Can you work these out from the model? Positions are in its coordinate system, mm. Face numbers are marked on the shaded views. Give positions to 0.01 mm unless a question says otherwise; leave off trailing zeros. Order: outer loops, then holes, each group sorted by start corner. A loop starts at its lowest first (then second) coordinate and runs counter-clockwise, first axis right, second up. Notation, with made-up numbers: M 9,1 L 37,1 A9 cw 37,16 Z; hole C 86,19 d6. An arc over 180 degrees is marked long. Answer as a JSON object with one key per item and string values.
```python
from build123d import *

# Parameters (mm, degrees)
SKETCH1_R                = 50
SKETCH1_R_2              = 2.778
BOSS_EXTRUDE1_DEPTH      = 2.5
SKETCH2_W                = 5
SKETCH2_H                = 63.3
BOSS_EXTRUDE2_DEPTH      = 50
FILLET1_R                = 10
SKETCH14_W               = 40.64
SKETCH14_H               = 20.32
CUT_EXTRUDE1_DEPTH       = 30.305745908
F_3_0_3_DIAMETER_HOLE1_D = 3
FILLET1_OF_MIRROR1_R     = 10


with BuildPart() as part:
    # Sketch1 → Boss-Extrude1 (new body, symmetric)
    with BuildSketch(Plane(origin=(0, 0, 0), x_dir=(1, 0, 0), z_dir=(0, 1, 0))):
        Circle(SKETCH1_R)
        Circle(SKETCH1_R_2, mode=Mode.SUBTRACT)
    extrude(amount=BOSS_EXTRUDE1_DEPTH, both=True)

    # Sketch2 → Boss-Extrude2 (add)
    with BuildSketch(Plane(origin=(0, 2.5, 0), x_dir=(1, 0, 0), z_dir=(0, 1, 0))):
        with Locations((-23.194254092, 0)):
            Rectangle(SKETCH2_W, SKETCH2_H)
    boss_extrude2 = extrude(amount=BOSS_EXTRUDE2_DEPTH)

    # Fillet1
    fillet1_edges = [part.edges().sort_by_distance(p)[0] for p in [
        (-23.194254092, 52.5, -31.65),
        (-23.194254092, 52.5, 31.65),
    ]]
    fillet(fillet1_edges, radius=FILLET1_R)

    # Sketch14 → Cut-Extrude1 (cut, through all)
    with BuildSketch(Plane(origin=(-20.694254092, 0, 0), x_dir=(0, 0, -1), z_dir=(1, 0, 0))):
        with Locations((-0.01, 32.34)):
            Rectangle(SKETCH14_W, SKETCH14_H)
        Polygon((-20.33, 31.705), (-20.33, 32.975), (-25.63, 32.975), (-25.63, 32.34), (-25.63, 31.705), align=None)
        Polygon((25.61, 32.975), (20.31, 32.975), (20.31, 31.705), (25.61, 31.705), (25.61, 32.34), align=None)
    cut_extrude1 = extrude(amount=-CUT_EXTRUDE1_DEPTH, mode=Mode.SUBTRACT)

    # Ø3.0 (3) Diameter Hole1 (through all)
    with Locations(Plane(origin=(-20.694254092, 0, 0), x_dir=(0, 0, -1), z_dir=(1, 0, 0))):
        with Locations((24.12, 37.42), (24.12, 27.26), (-24.14, 37.42), (-24.14, 27.26)):
            f_3_0_3_diameter_hole1 = Hole(F_3_0_3_DIAMETER_HOLE1_D / 2)

    # Mirror1: Boss-Extrude2, Cut-Extrude1, Ø3.0 (3) Diameter Hole1 across plane
    add(boss_extrude2.mirror(Plane(origin=(0, 0, 0), x_dir=(0, 0, 1), z_dir=(1, 0, 0))))
    add(cut_extrude1.mirror(Plane(origin=(0, 0, 0), x_dir=(0, 0, 1), z_dir=(1, 0, 0))), mode=Mode.SUBTRACT)
    add(f_3_0_3_diameter_hole1.mirror(Plane(origin=(0, 0, 0), x_dir=(0, 0, 1), z_dir=(1, 0, 0))), mode=Mode.SUBTRACT)

    # Fillet1 of Mirror1
    fillet1_of_mirror1_edges = [part.edges().sort_by_distance(p)[0] for p in [
        (23.194254092, 52.5, -31.65),
        (23.194254092, 52.5, 31.65),
    ]]
    fillet(fillet1_of_mirror1_edges, radius=FILLET1_OF_MIRROR1_R)


solid = part.part
```
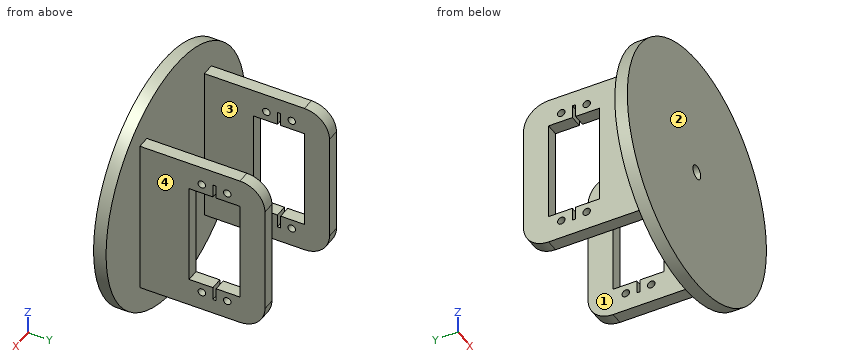
1) Thinking about a two-plate mould opening in X: for the marked faces 1, 2, 3 and 4, which applies, pulls with the +X half, pulls with the -X half, needs draft (parallel to the pull), parting line crosses it, or undercut?
Results found:
{"face 1": "undercut", "face 2": "needs draft", "face 3": "undercut", "face 4": "pulls with the +X half"}
2) I want a section at A-A on x = 0. Write out the boundary of the cut face in (y, z), and give its area (3 significant figures).
Results found:
{"outline": "M -2.5,-50 L 2.5,-50 L 2.5,-2.78 L -2.5,-2.78 Z; M -2.5,2.78 L 2.5,2.78 L 2.5,50 L -2.5,50 Z", "area": "472 mm²"}
3) I want a section at D-D on x = -23. Write out the boundary of the cut face in (y, z) (3 decimals), and give its area (3 significant figures).
Results found:
{"outline": "M -2.5,-44.396 L 2.5,-44.396 L 2.5,-31.65 L 42.5,-31.65 A10 ccw 52.5,-21.65 L 52.5,21.65 A10 ccw 42.5,31.65 L 2.5,31.65 L 2.5,44.396 L -2.5,44.396 Z; hole M 22.18,-20.31 L 31.705,-20.31 L 31.705,-25.61 L 32.975,-25.61 L 32.975,-20.31 L 42.5,-20.31 L 42.5,20.33 L 32.975,20.33 L 32.975,25.63 L 31.705,25.63 L 31.705,20.33 L 22.18,20.33 Z; hole C 27.26,-24.12 d3; hole C 27.26,24.14 d3; hole C 37.42,-24.12 d3; hole C 37.42,24.14 d3", "area": "2,700 mm²"}
4) I need wall thicknesses on L1, parallel to Z at x = 24.25, y = 37.42; L2, parallel to X at y = 46, z = -13; L3, parallel to Y at x = -21.9, z = -24.12 (3 decimals). Which ranges of each line are inside material? Lowest first, please.
Results found:
{"L1": "z = -31.65 to -25.62, -22.62 to -20.31, 20.33 to 22.64, 25.64 to 31.65", "L2": "x = -25.69 to -20.69, 20.69 to 25.69", "L3": "y = -2.5 to 25.76, 28.76 to 31.705, 32.975 to 35.92, 38.92 to 52.19"}
5) I want a section at C-C on z = 17. Write out the boundary of the cut face in (x, y), and give its area (3 significant figures).
Results found:
{"outline": "M -47.02,-2.5 L 47.02,-2.5 L 47.02,2.5 L 25.69,2.5 L 25.69,22.18 L 20.69,22.18 L 20.69,2.5 L -20.69,2.5 L -20.69,22.18 L -25.69,22.18 L -25.69,2.5 L -47.02,2.5 Z; M -25.69,42.5 L -20.69,42.5 L -20.69,52.5 L -25.69,52.5 Z; M 20.69,42.5 L 25.69,42.5 L 25.69,52.5 L 20.69,52.5 Z", "area": "767 mm²"}
6) I'm going to push flat-ended pins straight in: pin 1 Ø6 at (x, y) = (21.5, 32) entering from -Z; pin 2 Ø2.5 at (y, z) = (27.26, 24.14) entering from -X; pin 3 Ø3 at (x, z) = (-16, 9.5) entering from +Y; pin 4 Ø3.5 at (y, z) = (37.42, -24.12) entering from +X. Where does each tip first touch, or does it pass through?
Results found:
{"pin 1": "stops at z = -31.65", "pin 2": "passes through", "pin 3": "stops at y = 2.5", "pin 4": "stops at x = 25.69"}
7) I want a section at B-B on y = 27.26. Count the separate pieces of the cut face and the enclosed holes in it, and give its area (3 significant figures).
Results found:
{"separate pieces": "8", "enclosed holes": "0", "area": "167 mm²"}
